from build123d import *

# Parameters (mm, degrees)
BOSS_EXTRUDE1_DEPTH = 2.54


with BuildPart() as part:
    # Sketch1 → Boss-Extrude1 (new body)
    with BuildSketch(Plane.XY):
        with BuildLine():
            Line((0, 825.5), (0, 34.544))
            Line((0, 34.544), (15.24, 34.544))
            Line((15.24, 34.544), (15.24, 15.24))
            Line((15.24, 15.24), (34.544, 15.24))
            Line((34.544, 15.24), (34.544, 0))
            Line((34.544, 0), (627.60098, 0))
            ThreePointArc((627.60098, 0), (665.70098, 38.1), (703.80098, 0))
            Line((703.80098, 0), (872.45698, 0))
            Line((872.45698, 0), (872.45698, 15.24))
            Line((872.45698, 15.24), (891.76098, 15.24))
            Line((891.76098, 15.24), (891.76098, 34.544))
            Line((891.76098, 34.544), (907.00098, 34.544))
            Line((907.00098, 34.544), (907.00098, 825.5))
            Line((907.00098, 825.5), (0, 825.5))
        make_face()
    extrude(amount=BOSS_EXTRUDE1_DEPTH)


solid = part.part
Geometry check sheet. Reference: the model listing, model coordinates, mm. Give positions to 0.01 mm unless a question says otherwise; leave off trailing zeros.
1) Go/stop test with flat-tipped pins: pin 1 Ø1.3 at (y, z) = (28, 1.5) entering from +X; pin 2 Ø1.3 at (x, z) = (897.5, 1.5) entering from -Y; pin 3 Ø1.3 at (x, z) = (885, 1.5) entering from -Y. Record where each tip stops, or that it passes through.
Values follow:
pin 1: stops at x = 891.76
pin 2: stops at y = 34.54
pin 3: stops at y = 15.24
2) Thickness scan on line 1 (Y direction, x = 679.5, z = 0.95). Record the ranges inside material, lowest first.
Values follow:
line 1: y = 35.51 to 825.5
3) Release check for a two-part mould opening along X. For faces 1 (the face through (664.86, 38.09, 1.25)), 2 (the face through (447, 419, 2.54)) record: released by +X, released by -X, zero draft, split by the parting line, or undercut.
Values follow:
face 1: undercut
face 2: zero draft
